Input: part model. Units: mm. Frame: model coordinates. Face numbers are marked on the shaded views. Coordinates: 2 decimals unless noted, no trailing zeros. Order: outer loops, then holes, each group sorted by start corner. A loop starts at its lowest first (then second) coordinate and runs counter-clockwise, first axis right, second up. Notation, with made-up numbers: M 5.5,79 L 26.5,79 A35 cw 26.5,116 Z; hole C 31.5,-12 d1. An arc over 180 degrees is marked long. One line per item, written item: value.
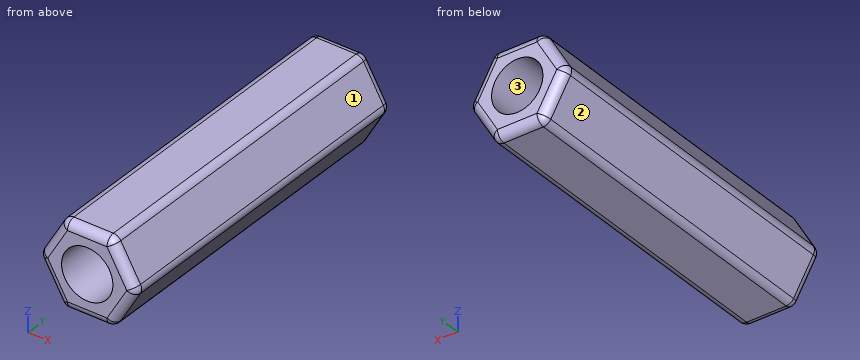
```python
from build123d import *

# Parameters (mm, degrees)
SKETCH1_R           = 1.5
BOSS_EXTRUDE1_DEPTH = 20
FILLET1_R           = 0.5


with BuildPart() as part:
    # Sketch1 → Boss-Extrude1 (new body)
    with BuildSketch(Plane(origin=(0, 0, 0), x_dir=(1, 0, 0), z_dir=(0, 1, 0))):
        Polygon((-1.443375673, 2.5), (-2.886751346, 0), (-1.443375673, -2.5), (1.443375673, -2.5), (2.886751346, 0), (1.443375673, 2.5), align=None)
        with Locations(Location((0, 0, 0), (0, 0, 270))):
            Circle(SKETCH1_R, mode=Mode.SUBTRACT)
    extrude(amount=BOSS_EXTRUDE1_DEPTH)

    # Fillet1
    fillet1_edges = [part.edges().sort_by_distance(p)[0] for p in [
        (-2.165063509, 20, 1.25),
        (1.443375673, 10, -2.5),
        (2.886751346, 10, 0),
        (1.443375673, 10, 2.5),
        (-1.443375673, 10, 2.5),
        (-2.886751346, 10, 0),
        (-1.443375673, 10, -2.5),
        (0, 20, 2.5),
        (2.165063509, 20, 1.25),
        (2.165063509, 20, -1.25),
        (0, 20, -2.5),
        (2.165063509, 0, -1.25),
        (2.165063509, 0, 1.25),
        (0, 0, 2.5),
        (-2.165063509, 20, -1.25),
        (-2.165063509, 0, 1.25),
        (-2.165063509, 0, -1.25),
        (0, 0, -2.5),
    ]]
    fillet(fillet1_edges, radius=FILLET1_R)


solid = part.part
```
(1) Cut plane A-A on x = -0.9. Output: boundary loops of the cut face in (y, z).
Data:
outline: M 0,-2 A0.5 ccw 0.5,-2.5 L 19.5,-2.5 A0.5 ccw 20,-2 L 20,-1.2 L 0,-1.2 Z; M 0,1.2 L 20,1.2 L 20,2 A0.5 ccw 19.5,2.5 L 0.5,2.5 A0.5 ccw 0,2 Z
(2) First-contact query: pin 1 (1 mm diameter, centred on x = -0.5, z = -0.5, fed in from -Y). Flat tip, straight axial feed; report the tip coordinate or a pass-through.
Data:
pin 1: passes through
(3) Ray query, line 1 (X direction, y = 14.5, z = 0); line 2 (Z direction, x = 1.55, y = 17.25); line 3 (X direction, y = 10.5, z = 0.3). Return the intervals inside material, ascending. Write a range as from..to.
Data:
line 1: x = -2.81..-1.5, 1.5..2.81
line 2: z = -2.31..2.31
line 3: x = -2.71..-1.47, 1.47..2.71
(4) Cut plane B-B on y = 9. Output: boundary loops of the cut face in (x, z), plus the area to 3 significant figures.
Data:
outline: M -2.74,-0.25 L -1.59,-2.25 A0.5 ccw -1.15,-2.5 L 1.15,-2.5 A0.5 ccw 1.59,-2.25 L 2.74,-0.25 A0.5 ccw 2.74,0.25 L 1.59,2.25 A0.5 ccw 1.15,2.5 L -1.15,2.5 A0.5 ccw -1.59,2.25 L -2.74,0.25 A0.5 ccw Z; hole C 0,0 d3
area: 14.5 mm2
(5) Cut plane C-C on x = 0. Output: boundary loops of the cut face in (y, z), plus the area to 3 significant figures.
Data:
outline: M 0,-2 A0.5 ccw 0.5,-2.5 L 19.5,-2.5 A0.5 ccw 20,-2 L 20,-1.5 L 0,-1.5 Z; M 0,1.5 L 20,1.5 L 20,2 A0.5 ccw 19.5,2.5 L 0.5,2.5 A0.5 ccw 0,2 Z
area: 39.8 mm2
(6) Draft query along Z for the marked faces 1, 2 and 3. Return one class per face: released by +Z, released by -Z, zero draft, split by the parting line, or undercut.
Data:
face 1: released by +Z
face 2: released by -Z
face 3: undercut
